from build123d import *

# Parameters (mm, degrees)
M10_TAPPED_HOLE1_D     = 8.5
M10_TAPPED_HOLE1_DEPTH = 24.5
M10_TAPPED_HOLE1_TIP   = 2.553657631


with BuildPart() as part:
    # Sketch1 → Revolve1 (revolve)
    with BuildSketch(Plane.XY, mode=Mode.PRIVATE) as revolve1_sk:
        Polygon((0, 0), (21, 0), (10, 9.5), (10, 19.5), (0, 19.5), align=None)
    revolve(revolve1_sk.sketch.rotate(Axis((0, 59.431666947, 0), (0, -1, 0)), 90), axis=Axis((0, 59.431666947, 0), (0, -1, 0)))

    # Sketch2 → Cut-Revolve1 (revolve, cut)
    with BuildSketch(Plane.XY, mode=Mode.PRIVATE) as cut_revolve1_sk:
        Polygon((0, 8), (10.971871481, 8), (20.235029376, 0), (0, 0), align=None)
    revolve(cut_revolve1_sk.sketch.rotate(Axis((0, 26.152643853, 0), (0, -1, 0)), 90), axis=Axis((0, 26.152643853, 0), (0, -1, 0)), mode=Mode.SUBTRACT)

    # M10 Tapped Hole1
    with Locations(Plane(origin=(0, 19.5, 0), x_dir=(1, 0, 0), z_dir=(0, 1, 0))):
        with Locations((0, 0)):
            Hole(M10_TAPPED_HOLE1_D / 2, depth=M10_TAPPED_HOLE1_DEPTH)
            with Locations((0, 0, -(M10_TAPPED_HOLE1_DEPTH + M10_TAPPED_HOLE1_TIP / 2))):  # 118° drill point
                Cone(0, M10_TAPPED_HOLE1_D / 2, M10_TAPPED_HOLE1_TIP, mode=Mode.SUBTRACT)


solid = part.part
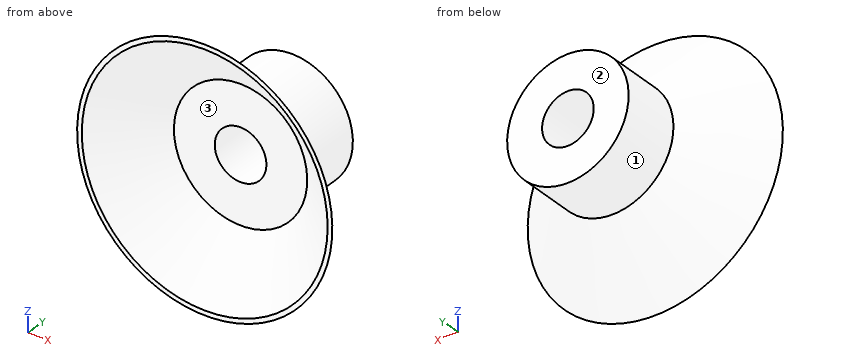
CAD build for the part. Positions are in the model's coordinates, mm. Face numbers are marked on the shaded views. Round coordinates to 2 decimals unless told otherwise and drop trailing zeros. Write each loop counter-clockwise with the first axis right and the second up, starting at its lowest first coordinate (ties: lowest second). Pieces come first, ordered by that corner, then holes. Notation, with made-up numbers: (38, -14) -> (61, -14) arc R22 cw to (61, 0) -> close; hole circle Ø3 at (-38, -17.75). An arc over 180 degrees is marked (long way). Answer as a JSON object with one key per item and string values.
(1) Band-saw the part on A-A, the plane z = 0. List the corners of the cut face in (x, y).
Reported:
{"outline": "(-21, 0) -> (-20.24, 0) -> (-10.97, 8) -> (-4.25, 8) -> (-4.25, 19.5) -> (-10, 19.5) -> (-10, 9.5) -> close; (4.25, 8) -> (10.97, 8) -> (20.24, 0) -> (21, 0) -> (10, 9.5) -> (10, 19.5) -> (4.25, 19.5) -> close"}
(2) Two-plate mould, pull along X, no slides. Class the marked faces 1, 2 and 3: +X half, -X half, draft (parallel to the pull), parting line (faces both ways), or undercut.
Reported:
{"face 1": "parting line", "face 2": "draft", "face 3": "undercut"}
(3) Probe probe 1 along X at (y, z) = (1, -11.5); probe 2 along Z at (x, y) = (-13, 1.75); probe 3 along Y at (x, z) = (7, 7). List the from-to ranges inside material, lowest first. Write a range as [from, to].
Reported:
{"probe 1": "x = [-16.17, -15.22], [15.22, 16.17]", "probe 2": "z = [-13.82, -12.75], [12.75, 13.82]", "probe 3": "y = [8, 19.5]"}
(4) Pin check, flat tips, straight feed: P1, Ø8, axis at y = 9, z = 3, coming from the +X side; P2, Ø5, axis at y = 7.5, z = 5, coming from the -X side; P3, Ø10, axis at x = 0, z = 0, coming from the -Y side; P4, Ø12, axis at x = -16.5, z = -16.5, coming from the -Y side. Stop position of each tip, or through.
Reported:
{"P1": "stops at x = 14.97", "P2": "stops at x = -14.47", "P3": "stops at y = 8", "P4": "stops at y = 0"}
(5) Band-saw the part on C-C, the plane y = 2.5. List the corners of the cut face in (x, z).
Reported:
{"outline": "circle Ø36.21 at (0, 0); hole circle Ø34.68 at (0, 0)"}
(6) Band-saw the part on B-B, the plane x = 0. List the corners of the cut face in (y, z), then the cut area to 3 significant figures.
Reported:
{"outline": "(0, -21) -> (9.5, -10) -> (19.5, -10) -> (19.5, -4.25) -> (8, -4.25) -> (8, -10.97) -> (0, -20.24) -> close; (0, 20.24) -> (8, 10.97) -> (8, 4.25) -> (19.5, 4.25) -> (19.5, 10) -> (9.5, 10) -> (0, 21) -> close", "area": "147 mm^2"}
